from build123d import *

# Parameters (mm, degrees)
ESBO_O1_R                = 1.5
RESSALTO_EXTRUS_O1_DEPTH = 2.5


with BuildPart() as part:
    # Esboço1 → Ressalto-extrusão1 (new body)
    with BuildSketch(Plane.XY):
        with BuildLine():
            Line((-10, 3), (-7.9, 3))
            Line((-7.9, 3), (-7.9, 6.5))
            Line((-7.9, 6.5), (7.9, 6.5))
            Line((7.9, 6.5), (7.9, 3))
            Line((7.9, 3), (10, 3))
            ThreePointArc((10, 3), (13, 0), (10, -3))
            Line((10, -3), (7.9, -3))
            Line((7.9, -3), (7.9, -6.5))
            Line((7.9, -6.5), (-7.9, -6.5))
            Line((-7.9, -6.5), (-7.9, -3))
            Line((-7.9, -3), (-10, -3))
            ThreePointArc((-10, -3), (-13, 0), (-10, 3))
        make_face()
        with Locations((-10, 0)):
            Circle(ESBO_O1_R, mode=Mode.SUBTRACT)
        with Locations((10, 0)):
            Circle(ESBO_O1_R, mode=Mode.SUBTRACT)
    extrude(amount=RESSALTO_EXTRUS_O1_DEPTH)


solid = part.part
Source: CAD feature listing. Evaluate the final solid. Frame: model axes, mm. A direction names the side the tool comes from. Coordinates: 2 decimals unless noted, no trailing zeros. Write each loop counter-clockwise with the first axis right and the second up, starting at its lowest first coordinate (ties: lowest second). Pieces come first, ordered by that corner, then holes. Notation, with made-up numbers: M 77,-6 L 94,-6 A4 cw 94,0 Z; hole C -10,38.5 d11. An arc over 180 degrees is marked long. Use a Markdown table: item, result.
1) Ray query, L1, parallel to Y at x = -10, z = 1.8; L2, parallel to X at y = 4.5, z = 0.8; L3, parallel to Y at x = -11, z = 1.45. Return the intervals inside material, ascending.
Conclusion:
| item | result |
|---|---|
| L1 | y = -3 to -1.5, 1.5 to 3 |
| L2 | x = -7.9 to 7.9 |
| L3 | y = -2.83 to -1.12, 1.12 to 2.83 |
2) First-contact query: pin 1 Ø1 at (x, z) = (-9, 1) entering from +Y; pin 2 Ø1.2 at (y, z) = (-4, 2) entering from +X; pin 3 Ø0.8 at (y, z) = (-4.5, 0.5) entering from -X. Flat tips, straight axial feed; report the tip coordinate or a pass-through.
Conclusion:
| item | result |
|---|---|
| pin 1 | stops at y = 3 |
| pin 2 | stops at x = 7.9 |
| pin 3 | stops at x = -7.9 |
3) Section C-C, the plane y = -3.5. Output: boundary loops of the cut face in (x, z), then the cut area to 3 significant figures.
Conclusion:
| item | result |
|---|---|
| outline | M -7.9,0 L 7.9,0 L 7.9,2.5 L -7.9,2.5 Z |
| area | 39.5 mm^2 |
4) Section D-D, the plane y = 2. Output: boundary loops of the cut face in (x, z), then the cut area to 3 significant figures.
Conclusion:
| item | result |
|---|---|
| outline | M -12.24,0 L 12.24,0 L 12.24,2.5 L -12.24,2.5 Z |
| area | 61.2 mm^2 |
5) Section B-B, the plane y = 0. Output: boundary loops of the cut face in (x, z).
Conclusion:
| item | result |
|---|---|
| outline | M -13,0 L -11.5,0 L -11.5,2.5 L -13,2.5 Z; M -8.5,0 L 8.5,0 L 8.5,2.5 L -8.5,2.5 Z; M 11.5,0 L 13,0 L 13,2.5 L 11.5,2.5 Z |
6) Section A-A, the plane z = 1.75. Output: boundary loops of the cut face in (x, y).
Conclusion:
| item | result |
|---|---|
| outline | M -10,-3 L -7.9,-3 L -7.9,-6.5 L 7.9,-6.5 L 7.9,-3 L 10,-3 A3 ccw 10,3 L 7.9,3 L 7.9,6.5 L -7.9,6.5 L -7.9,3 L -10,3 A3 ccw Z; hole C -10,0 d3; hole C 10,0 d3 |
7) Reachability of faces 5 (the flat face through (-9, 3, 1)), 6 (the flat face through (-9, -3, 1)), 7 (the flat face through (9, -3, 1)) from +Z, -Z, +X, -X, +Y, -Y: full face, straight path, thin tool, end or side. Return the list, or none.
Conclusion:
| item | result |
|---|---|
| face 5 | +Z, -Z, -X, +Y |
| face 6 | +Z, -Z, -X, -Y |
| face 7 | +Z, -Z, +X, -Y |
8) Mould query, pull axis X, two halves, no side actions, for faces 1 (the flat face through (0, 0, 2.5)), 2 (the cylindrical face through (-13, 0, 1)), 3 (the flat face through (7.9, 5, 1)), 4 (the cylindrical face through (-11.5, 0.07, 1.23)). Classes: pulls with the +X half, pulls with the -X half, needs draft (parallel to the pull), parting line crosses it, or undercut.
Conclusion:
| item | result |
|---|---|
| face 1 | needs draft |
| face 2 | pulls with the -X half |
| face 3 | pulls with the +X half |
| face 4 | undercut |
